```python
from build123d import *

# Parameters (mm, degrees)
BASE_FLANGE1_DEPTH           = 2
EDGE_FLANGE1_STRIP_W         = 9.4732
EDGE_FLANGE1_STRIP_H         = 2
EDGE_FLANGE1_STRIP_CUT_DEPTH = 65
EDGE_FLANGE1_DEPTH           = 65
EDGE_FLANGE2_STRIP_W         = 9.4732
EDGE_FLANGE2_STRIP_H         = 2
EDGE_FLANGE2_STRIP_CUT_DEPTH = 65
EDGE_FLANGE2_DEPTH           = 65


# Sheet-metal steps are written as plain solids
with BuildPart() as part:
    # Sketch1 → Base-Flange1 (new body)
    with BuildSketch(Plane.XY):
        Polygon((-80, 206), (-80, 36), (-112.26, 16), (-112.26, -34), (-80, -34), (-80, -38), (-15, -38), (-15, -34), (15, -34), (15, -38), (80, -38), (80, -34), (112.26, -34), (112.26, 16), (80, 36), (80, 206), align=None)
        with BuildLine():
            Line((-110.26, -6), (-110.26, 6))
            ThreePointArc((-110.26, 6), (-108.16, 8.1), (-106.06, 6))
            Line((-106.06, 6), (-106.06, -6))
            ThreePointArc((-106.06, -6), (-108.16, -8.1), (-110.26, -6))
        make_face(mode=Mode.SUBTRACT)
        with BuildLine():
            Line((106.06, -6), (106.06, 6))
            ThreePointArc((106.06, 6), (108.16, 8.1), (110.26, 6))
            Line((110.26, 6), (110.26, -6))
            ThreePointArc((110.26, -6), (108.16, -8.1), (106.06, -6))
        make_face(mode=Mode.SUBTRACT)
    extrude(amount=-BASE_FLANGE1_DEPTH)

    # Edge-Flange1 strip (across the edge) → Edge-Flange1 strip cut (cut)
    with BuildSketch(Plane(origin=(-80, -38, 0), x_dir=(0, 1, 0), z_dir=(1, 0, 0))):
        with Locations((-2, -1)):
            Rectangle(EDGE_FLANGE1_STRIP_W, EDGE_FLANGE1_STRIP_H)
    extrude(amount=EDGE_FLANGE1_STRIP_CUT_DEPTH, mode=Mode.SUBTRACT)

    # Edge-Flange1 section (across the edge) → Edge-Flange1 (add)
    with BuildSketch(Plane(origin=(-80, -38, 0), x_dir=(0, 1, 0), z_dir=(1, 0, 0))):
        with BuildLine():
            Line((0, 0.7366), (0, 18))
            Line((0, 18), (2, 18))
            Line((2, 18), (2, 0.7366))
            ThreePointArc((2, 0.7366), (2.215745145, 0.215745145), (2.7366, 0))
            Line((2.7366, 0), (2.7366, -2))
            ThreePointArc((2.7366, -2), (0.801531583, -1.198468417), (0, 0.7366))
        make_face()
    extrude(amount=EDGE_FLANGE1_DEPTH)

    # Edge-Flange2 strip (across the edge) → Edge-Flange2 strip cut (cut)
    with BuildSketch(Plane(origin=(80, -38, -2), x_dir=(0, 1, 0), z_dir=(-1, 0, 0))):
        with Locations((-2, -1)):
            Rectangle(EDGE_FLANGE2_STRIP_W, EDGE_FLANGE2_STRIP_H)
    extrude(amount=EDGE_FLANGE2_STRIP_CUT_DEPTH, mode=Mode.SUBTRACT)

    # Edge-Flange2 section (across the edge) → Edge-Flange2 (add)
    with BuildSketch(Plane(origin=(80, -38, -2), x_dir=(0, 1, 0), z_dir=(-1, 0, 0))):
        with BuildLine():
            Line((0, 0.7366), (0, 18))
            Line((0, 18), (2, 18))
            Line((2, 18), (2, 0.7366))
            ThreePointArc((2, 0.7366), (2.215745145, 0.215745145), (2.7366, 0))
            Line((2.7366, 0), (2.7366, -2))
            ThreePointArc((2.7366, -2), (0.801531583, -1.198468417), (0, 0.7366))
        make_face()
    extrude(amount=EDGE_FLANGE2_DEPTH)


solid = part.part
```
Geometry: final body of the model. Coordinates: model frame, mm. A direction names the side the tool comes from. Coordinates: 2 decimals unless noted, no trailing zeros. Order: outer loops, then holes, each group sorted by start corner. A loop starts at its lowest first (then second) coordinate and runs counter-clockwise, first axis right, second up. Notation, with made-up numbers: (6, -30) - (35, -30) arc R18 cw to (35, -17) - close; hole circle Ø6 at (59.25, -28). An arc over 180 degrees is marked (long way). Return JSON: item names as keys, results as strings. Group by question number.
1. Pin query (flat end, axial travel): pin 1 (4.5 mm diameter, centred on y = -35, z = -14, fed in from -X); pin 2 (0.6 mm diameter, centred on y = 120, z = -1, fed in from -X); pin 3 (12 mm diameter, centred on y = 36.5, z = -0.5, fed in from -X); pin 4 (10 mm diameter, centred on x = -11.5, z = -1.5, fed in from -Y). Return the tip coordinate at first contact, or that it passes through.
2. Material intervals for line 1 along Z through (x, y) = (-8, 180); line 2 along Y through (x, z) = (48, -18); line 3 along Y through (x, z) = (93, -1), sorted ascending. Write a range as [from, to].
3. Cut plane C-C (z = -16). Output: boundary loops of the cut face in (x, y), plus the area to 3 significant figures.
4. Cut plane B-B (y = 182). Output: boundary loops of the cut face in (x, z), plus the area to 3 significant figures.
5. Set-up query: faces 1 (the face through (48, -38, -11)), 2 (the face through (48, -36, -11)), 3 (the face through (-48, -36, 9)). Return all of +Z, -Z, +X, -X, +Y, -Y with unobstructed straight access to the full face (end or side cutting, diameter ignored); none if empty.
6. Cut plane A-A (x = -27). Output: boundary loops of the cut face in (y, z), plus the area to 3 significant figures.
Resolved:
{
 "1": {"pin 1": "stops at x = 15", "pin 2": "stops at x = -80", "pin 3": "stops at x = -88.87", "pin 4": "stops at y = -38"},
 "2": {"line 1": "z = [-2, 0]", "line 2": "y = [-38, -36]", "line 3": "y = [-34, 27.94]"},
 "3": {"outline": "(15, -38) - (80, -38) - (80, -36) - (15, -36) - close", "area": "130 mm²"},
 "4": {"outline": "(-80, -2) - (80, -2) - (80, 0) - (-80, 0) - close", "area": "320 mm²"},
 "5": {"face 1": "+Z, -Z, +X, -X, -Y", "face 2": "-Z, +X, -X, +Y", "face 3": "+Z, +X, -X, +Y"},
 "6": {"outline": "(-38, 0.74) arc R2.74 ccw to (-35.26, -2) - (206, -2) - (206, 0) - (-35.26, 0) arc R0.74 cw to (-36, 0.74) - (-36, 18) - (-38, 18) - close", "area": "523 mm²"}
}
